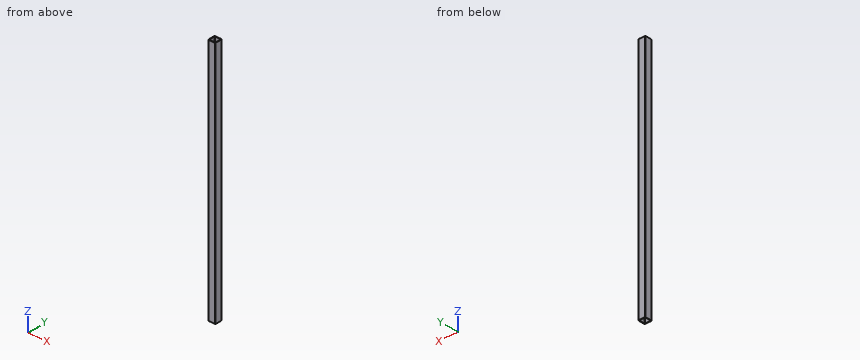
from build123d import *

# Parameters (mm, degrees)
BOSS_EXTRUDE1_DEPTH     = 1500
CUT_EXTRUDE3_DEPTH      = 1501.967428028
CUT_EXTRUDE3_DEPTH_BACK = 1501.967428028
SKETCH2_W               = 432.224270186
SKETCH2_H               = 1076.950896283
SKETCH2_W_2             = 908.538956416
SKETCH2_H_2             = 1717.469993805


with BuildPart() as part:
    # Sketch1 → Boss-Extrude1 (new body)
    with BuildSketch(Plane.XY):
        with BuildLine():
            Line((2.54, 0), (35.56, 0))
            ThreePointArc((35.56, 0), (37.356051224, -0.743948776), (38.1, -2.54))
            Line((38.1, -2.54), (38.1, -35.56))
            ThreePointArc((38.1, -35.56), (37.356051224, -37.356051224), (35.56, -38.1))
            Line((35.56, -38.1), (2.54, -38.1))
            ThreePointArc((2.54, -38.1), (0.743948776, -37.356051224), (0, -35.56))
            Line((0, -35.56), (0, -2.54))
            ThreePointArc((0, -2.54), (0.743948776, -0.743948776), (2.54, 0))
        make_face()
        with BuildLine():
            Line((5.3086, -2.7686), (32.7914, -2.7686))
            ThreePointArc((32.7914, -2.7686), (34.587451224, -3.512548776), (35.3314, -5.3086))
            Line((35.3314, -5.3086), (35.3314, -32.7914))
            ThreePointArc((35.3314, -32.7914), (34.587451224, -34.587451224), (32.7914, -35.3314))
            Line((32.7914, -35.3314), (5.3086, -35.3314))
            ThreePointArc((5.3086, -35.3314), (3.512548776, -34.587451224), (2.7686, -32.7914))
            Line((2.7686, -32.7914), (2.7686, -5.3086))
            ThreePointArc((2.7686, -5.3086), (3.512548776, -3.512548776), (5.3086, -2.7686))
        make_face(mode=Mode.SUBTRACT)
    extrude(amount=BOSS_EXTRUDE1_DEPTH)

    # Sketch2 → Cut-Extrude3 (cut, two sides: drawn at the far end of the back side and taken through both)
    with BuildSketch(Plane.ZY.offset(-CUT_EXTRUDE3_DEPTH_BACK)):
        with Locations((-216.112135093, 500.375448142)):
            Rectangle(SKETCH2_W, SKETCH2_H)
        with Locations((1751.205155953, -66.993484906)):
            Rectangle(SKETCH2_W_2, SKETCH2_H_2)
    extrude(amount=CUT_EXTRUDE3_DEPTH + CUT_EXTRUDE3_DEPTH_BACK, mode=Mode.SUBTRACT)


solid = part.part
Source: CAD feature listing. Evaluate the final solid. Frame: model axes, mm. Round coordinates to 2 decimals unless told otherwise and drop trailing zeros. Loops run counter-clockwise (first coordinate to the right, second up) from the corner with the lowest first, then second, coordinate; pieces in that order, holes last. Notation, with made-up numbers: M -18,33 L 2,33 A32 ccw 2,72 Z; hole C -16.75,2 d6. An arc over 180 degrees is marked long. Return JSON: item names as keys, results as strings. Group by question number.
1. Section query B-B on y = -27. Output: boundary loops of the cut face in (x, z).
2. Material intervals for line 1 along Y through (x, z) = (14, 662.5); line 2 along X through (y, z) = (-9.5, 783); line 3 along Y through (x, z) = (3, 631), sorted ascending. Write a range as from..to.
3. Section query C-C on z = 310.5. Output: boundary loops of the cut face in (x, y), and give its area (3 significant figures).
4. Section query A-A on x = 11.5. Output: boundary loops of the cut face in (y, z), and give its area (3 significant figures).
Checks:
{
 "1": {"outline": "M 0,0 L 2.77,0 L 2.77,1296.94 L 0,1296.94 Z; M 35.33,0 L 38.1,0 L 38.1,1296.94 L 35.33,1296.94 Z"},
 "2": {"line 1": "y = -38.1..-35.33, -2.77..0", "line 2": "x = 0..2.77, 35.33..38.1", "line 3": "y = -38.1..-33.85, -4.25..0"},
 "3": {"outline": "M 0,-35.56 A2.54 ccw 2.54,-38.1 L 35.56,-38.1 A2.54 ccw 38.1,-35.56 L 38.1,-2.54 A2.54 ccw 35.56,0 L 2.54,0 A2.54 ccw 0,-2.54 Z; hole M 2.77,-32.79 A2.54 ccw 5.31,-35.33 L 32.79,-35.33 A2.54 ccw 35.33,-32.79 L 35.33,-5.31 A2.54 ccw 32.79,-2.77 L 5.31,-2.77 A2.54 ccw 2.77,-5.31 Z", "area": "391 mm²"},
 "4": {"outline": "M -38.1,0 L -35.33,0 L -35.33,1296.94 L -38.1,1296.94 Z; M -2.77,0 L 0,0 L 0,1296.94 L -2.77,1296.94 Z", "area": "7,180 mm²"}
}
